Geometry: final body of the model. Coordinates: model frame, mm. Coordinates: 2 decimals unless noted, no trailing zeros. Loops run counter-clockwise (first coordinate to the right, second up) from the corner with the lowest first, then second, coordinate; pieces in that order, holes last. Notation, with made-up numbers: (71, 29) - (125, 29) arc R16 cw to (125, 36) - close; hole circle Ø4 at (-5, 83). An arc over 180 degrees is marked (long way). Put each result on its own line as item: value. Start each with the question number.
1) Material intervals for line 1 along Y through (x, z) = (0, 0.8); line 2 along X through (y, z) = (-8.5, 0.65); line 3 along Y through (x, z) = (2.5, 0.2), sorted ascending. Write a range as from..to.
2) Section C-C on x = -12. Output: boundary loops of the cut face in (y, z), and give its area (3 significant figures).
3) Contact query for a flat-ended pin moving along its axis: pin 1 Ø4 at (x, y) = (21.43, -12.38) entering from -Z. Output: stop coordinate, or through.
4) Section D-D on z = 0.45. Output: boundary loops of the cut face in (x, y) (3 decimals), and give its area (3 significant figures).
5) Draft query along X for faces 1 (the cylindrical face through (-4.336, -19.524, 0.74)), 2 (the flat face through (-7, 19, 1.5)), 3 (the cylindrical face through (15.19, 23.82, 0.74)). Return one class per face: +X half, -X half, draft (parallel to the pull), parting line (faces both ways), or undercut.
6) Section B-B on x = 0. Output: boundary loops of the cut face in (y, z), and give its area (4 significant figures).
7) Section A-A on y = 0. Output: boundary loops of the cut face in (x, z).
```python
from build123d import *

# Parameters (mm, degrees)
SKETCH_1_R          = 28.25
SKETCH_1_R_2        = 20
EXTRUDE_1_DEPTH     = 1.5
SKETCH_2_R          = 1.6
CUT_EXTRUDE_1_DEPTH = 1.5


with BuildPart() as part:
    # 草图1 → 凸台-拉伸1 (new body)
    with BuildSketch(Plane.XY):
        Circle(SKETCH_1_R)
        Circle(SKETCH_1_R_2, mode=Mode.SUBTRACT)
    extrude(amount=EXTRUDE_1_DEPTH)

    # 草图2 → 切除-拉伸1 (cut)
    with BuildSketch(Plane.XY.offset(1.5)):
        with Locations((0, 24.75)):
            Circle(SKETCH_2_R)
        with Locations((21.434128744, 12.375)):
            Circle(SKETCH_2_R)
        with Locations((21.434128744, -12.375)):
            Circle(SKETCH_2_R)
        with Locations((0, -24.75)):
            Circle(SKETCH_2_R)
        with Locations((-21.434128744, -12.375)):
            Circle(SKETCH_2_R)
        with Locations((-21.434128744, 12.375)):
            Circle(SKETCH_2_R)
    extrude(amount=-CUT_EXTRUDE_1_DEPTH, mode=Mode.SUBTRACT)


solid = part.part
```
Answer block:
1. line 1: y = -28.25..-26.35, -23.15..-20, 20..23.15, 26.35..28.25
1. line 2: x = -26.94..-18.1, 18.1..26.94
1. line 3: y = -28.14..-19.84, 19.84..28.14
2. outline: (-25.57, 0) - (-16, 0) - (-16, 1.5) - (-25.57, 1.5) - close; (16, 0) - (25.57, 0) - (25.57, 1.5) - (16, 1.5) - close
2. area: 28.7 mm²
3. pin 1: stops at z = 0
4. outline: circle Ø56.5 at (0, 0); hole circle Ø3.2 at (-21.434, -12.375); hole circle Ø3.2 at (-21.434, 12.375); hole circle Ø40 at (0, 0); hole circle Ø3.2 at (0, -24.75); hole circle Ø3.2 at (0, 24.75); hole circle Ø3.2 at (21.434, -12.375); hole circle Ø3.2 at (21.434, 12.375)
4. area: 1,200 mm²
5. face 1: undercut
5. face 2: draft
5. face 3: parting line
6. outline: (-28.25, 0) - (-26.35, 0) - (-26.35, 1.5) - (-28.25, 1.5) - close; (-23.15, 0) - (-20, 0) - (-20, 1.5) - (-23.15, 1.5) - close; (20, 0) - (23.15, 0) - (23.15, 1.5) - (20, 1.5) - close; (26.35, 0) - (28.25, 0) - (28.25, 1.5) - (26.35, 1.5) - close
6. area: 15.15 mm²
7. outline: (-28.25, 0) - (-20, 0) - (-20, 1.5) - (-28.25, 1.5) - close; (20, 0) - (28.25, 0) - (28.25, 1.5) - (20, 1.5) - close
